Model file for the job. Use its own axes, mm. A direction names the side the tool comes from. Coordinates: 2 decimals unless noted, no trailing zeros. Return JSON: item names as keys, results as strings.
```python
from build123d import *

# Parameters (mm, degrees)
SKETCH1_R           = 1.5875
SKETCH1_W           = 0.7493
SKETCH1_H           = 15.875
BOSS_EXTRUDE1_DEPTH = 3.175


with BuildPart() as part:
    # Sketch1 → Boss-Extrude1 (new body)
    with BuildSketch(Plane.XY.offset(-676.275)):
        with BuildLine():
            Line((94.488, -171.45), (94.488, -136.525))
            Line((94.488, -136.525), (88.9, -136.525))
            Line((88.9, -136.525), (88.9, -111.125))
            Line((88.9, -111.125), (94.488, -111.125))
            Line((94.488, -111.125), (94.488, -85.725))
            Line((94.488, -85.725), (88.9, -85.725))
            Line((88.9, -85.725), (88.9, -60.325))
            Line((88.9, -60.325), (94.488, -60.325))
            Line((94.488, -60.325), (94.488, -25.4))
            ThreePointArc((94.488, -25.4), (87.271696875, -7.978303125), (69.85, -0.762))
            Line((69.85, -0.762), (-69.85, -0.762))
            ThreePointArc((-69.85, -0.762), (-87.271696875, -7.978303125), (-94.488, -25.4))
            Line((-94.488, -25.4), (-94.488, -60.325))
            Line((-94.488, -60.325), (-88.9, -60.325))
            Line((-88.9, -60.325), (-88.9, -85.725))
            Line((-88.9, -85.725), (-94.488, -85.725))
            Line((-94.488, -85.725), (-94.488, -111.125))
            Line((-94.488, -111.125), (-88.9, -111.125))
            Line((-88.9, -111.125), (-88.9, -136.525))
            Line((-88.9, -136.525), (-94.488, -136.525))
            Line((-94.488, -136.525), (-94.488, -171.45))
            ThreePointArc((-94.488, -171.45), (-87.271696875, -188.871696875), (-69.85, -196.088))
            Line((-69.85, -196.088), (69.85, -196.088))
            ThreePointArc((69.85, -196.088), (87.271696875, -188.871696875), (94.488, -171.45))
        make_face()
        with Locations(Location((63.1655201, -139.7, 0), (0, 0, 180))):
            Circle(SKETCH1_R, mode=Mode.SUBTRACT)
        with Locations(Location((-63.1655201, -51.5992872, 0), (0, 0, 180))):
            Circle(SKETCH1_R, mode=Mode.SUBTRACT)
        with Locations(Location((25.4, -183.388, 0), (0, 0, 180))):
            Circle(SKETCH1_R, mode=Mode.SUBTRACT)
        with Locations(Location((-25.4, -183.388, 0), (0, 0, 180))):
            Circle(SKETCH1_R, mode=Mode.SUBTRACT)
        with Locations(Location((-63.1655201, -139.7, 0), (0, 0, 180))):
            Circle(SKETCH1_R, mode=Mode.SUBTRACT)
        with Locations(Location((63.1655201, -51.5992872, 0), (0, 0, 180))):
            Circle(SKETCH1_R, mode=Mode.SUBTRACT)
        with BuildLine():
            Line((7.264641701, -112.328307791), (43.598023874, -137.666473794))
            ThreePointArc((43.598023874, -137.666473794), (46.023616914, -144.778727737), (39.965703023, -149.225))
            Line((39.965703023, -149.225), (-39.965703023, -149.225))
            ThreePointArc((-39.965703023, -149.225), (-46.023616914, -144.778727737), (-43.598023874, -137.666473794))
            Line((-43.598023874, -137.666473794), (-7.264641701, -112.328307791))
            ThreePointArc((-7.264641701, -112.328307791), (0, -110.045360203), (7.264641701, -112.328307791))
        make_face(mode=Mode.SUBTRACT)
        with BuildLine():
            Line((39.04526783, -56.807813406), (3.632320851, -81.504086518))
            ThreePointArc((3.632320851, -81.504086518), (0, -82.645560312), (-3.632320851, -81.504086518))
            Line((-3.632320851, -81.504086518), (-39.04526783, -56.807813406))
            ThreePointArc((-39.04526783, -56.807813406), (-41.47086087, -49.695559463), (-35.41294698, -45.2492872))
            Line((-35.41294698, -45.2492872), (35.41294698, -45.2492872))
            ThreePointArc((35.41294698, -45.2492872), (41.47086087, -49.695559463), (39.04526783, -56.807813406))
        make_face(mode=Mode.SUBTRACT)
        with BuildLine():
            Line((69.85, -70.72011097), (69.85, -92.075))
            ThreePointArc((69.85, -92.075), (67.990128061, -96.565128061), (63.5, -98.425))
            Line((63.5, -98.425), (27.826758339, -98.425))
            ThreePointArc((27.826758339, -98.425), (23.283322921, -95.090295803), (25.102517701, -89.756105345))
            Line((25.102517701, -89.756105345), (59.867679149, -65.511584764))
            ThreePointArc((59.867679149, -65.511584764), (66.4374532, -65.090380186), (69.85, -70.72011097))
        make_face(mode=Mode.SUBTRACT)
        with BuildLine():
            Line((-59.867679149, -65.511584764), (-25.102517701, -89.756105345))
            ThreePointArc((-25.102517701, -89.756105345), (-23.283322921, -95.090295803), (-27.826758339, -98.425))
            Line((-27.826758339, -98.425), (-63.5, -98.425))
            ThreePointArc((-63.5, -98.425), (-67.990128061, -96.565128061), (-69.85, -92.075))
            Line((-69.85, -92.075), (-69.85, -70.72011097))
            ThreePointArc((-69.85, -70.72011097), (-66.4374532, -65.090380186), (-59.867679149, -65.511584764))
        make_face(mode=Mode.SUBTRACT)
        with BuildLine():
            Line((-69.85, -186.563), (-34.925, -186.563))
            ThreePointArc((-34.925, -186.563), (-32.67993597, -185.63306403), (-31.75, -183.388))
            Line((-31.75, -183.388), (-31.75, -174.625))
            ThreePointArc((-31.75, -174.625), (-32.67993597, -172.37993597), (-34.925, -171.45))
            Line((-34.925, -171.45), (-79.039746678, -171.45))
            ThreePointArc((-79.039746678, -171.45), (-83.108999442, -173.738113573), (-83.268157726, -178.403834356))
            ThreePointArc((-83.268157726, -178.403834356), (-77.702052928, -184.363095439), (-69.85, -186.563))
        make_face(mode=Mode.SUBTRACT)
        with BuildLine():
            Line((69.85, -10.287), (-69.85, -10.287))
            ThreePointArc((-69.85, -10.287), (-78.244855824, -12.833012903), (-83.811231367, -19.613223028))
            ThreePointArc((-83.811231367, -19.613223028), (-83.371868677, -24.08222496), (-79.411683667, -26.1992872))
            Line((-79.411683667, -26.1992872), (79.411683667, -26.1992872))
            ThreePointArc((79.411683667, -26.1992872), (83.371868677, -24.08222496), (83.811231367, -19.613223028))
            ThreePointArc((83.811231367, -19.613223028), (78.244855824, -12.833012903), (69.85, -10.287))
        make_face(mode=Mode.SUBTRACT)
        with BuildLine():
            Line((-19.05, -183.388), (-19.05, -174.625))
            ThreePointArc((-19.05, -174.625), (-18.12006403, -172.37993597), (-15.875, -171.45))
            Line((-15.875, -171.45), (15.875, -171.45))
            ThreePointArc((15.875, -171.45), (18.12006403, -172.37993597), (19.05, -174.625))
            Line((19.05, -174.625), (19.05, -183.388))
            ThreePointArc((19.05, -183.388), (18.12006403, -185.63306403), (15.875, -186.563))
            Line((15.875, -186.563), (-15.875, -186.563))
            ThreePointArc((-15.875, -186.563), (-18.12006403, -185.63306403), (-19.05, -183.388))
        make_face(mode=Mode.SUBTRACT)
        with BuildLine():
            Line((31.75, -174.625), (31.75, -183.388))
            ThreePointArc((31.75, -183.388), (32.67993597, -185.63306403), (34.925, -186.563))
            Line((34.925, -186.563), (69.85, -186.563))
            ThreePointArc((69.85, -186.563), (77.702052928, -184.363095439), (83.268157726, -178.403834356))
            ThreePointArc((83.268157726, -178.403834356), (83.108999442, -173.738113573), (79.039746678, -171.45))
            Line((79.039746678, -171.45), (34.925, -171.45))
            ThreePointArc((34.925, -171.45), (32.67993597, -172.37993597), (31.75, -174.625))
        make_face(mode=Mode.SUBTRACT)
        with Locations((-89.27465, -153.9875)):
            Rectangle(SKETCH1_W, SKETCH1_H, mode=Mode.SUBTRACT)
        with Locations((89.27465, -153.9875)):
            Rectangle(SKETCH1_W, SKETCH1_H, mode=Mode.SUBTRACT)
    extrude(amount=-BOSS_EXTRUDE1_DEPTH)


solid = part.part
```
Item 1: Pull direction Y, two halves, no side cores. Call faces 3 (the flat face through (-25.686, -125.175, -677.84)), 4 (the flat face through (-1, -97, -676.275)), 5 (the cylindrical face through (-87.46, -188.68, -677.84)): +Y half, -Y half, draft (parallel to the pull), parting line (faces both ways), or undercut.
Check result:
{"face 3": "undercut", "face 4": "draft", "face 5": "-Y half"}
Item 2: 3-axis set-ups, long thin cutter, end or side, ignore diameter. For faces 1 (the cylindrical face through (-83.408, -24.028, -677.84)), 2 (the flat face through (-1, -97, -679.45)): which of +Z, -Z, +X, -X, +Y, -Y reach the whole face in a straight line?
Check result:
{"face 1": "+Z, -Z", "face 2": "-Z, +X, -X, +Y, -Y"}
Item 3: Wall check: line 1 (X direction, y = -152, z = -677.7); line 2 (X direction, y = -181, z = -676.55); line 3 (Y direction, x = -10, z = -676.7) (3 decimals). Give the ranges that are in metal, low to high.
Check result:
{"line 1": "x = -94.49 to -89.65, -88.9 to 88.9, 89.65 to 94.49", "line 2": "x = -92.56 to -81.56, -31.75 to -19.05, 19.05 to 31.75, 81.56 to 92.56", "line 3": "y = -196.088 to -186.563, -171.45 to -149.225, -114.236 to -77.063, -45.249 to -26.199, -10.287 to -0.762"}
Item 4: Drop flat-ended pins along their axis: pin 1 Ø2 at (x, y) = (-38.5, -97) entering from +Z; pin 2 Ø1 at (y, z) = (-79.5, -678) entering from +X; pin 3 Ø1 at (y, z) = (-82.5, -677.5) entering from -X. Give the stop position or say it passes through.
Check result:
{"pin 1": "passes through", "pin 2": "stops at x = 88.9", "pin 3": "stops at x = -88.9"}
Item 5: Saw through at A-A (z = -677.55). Count the separate pieces of the cut face and the enclosed holes in it, and give its area (3 significant figures).
Check result:
{"separate pieces": "1", "enclosed holes": "16", "area": "24,600 mm2"}
